Work out the finished part from the listing and answer in its coordinate system (mm). A direction names the side the tool comes from. Round coordinates to 2 decimals unless told otherwise and drop trailing zeros. Write each loop counter-clockwise with the first axis right and the second up, starting at its lowest first coordinate (ties: lowest second). Pieces come first, ordered by that corner, then holes.
from build123d import *

# Parameters (mm, degrees)
F0_R     = 1.6
F1_DEPTH = 7.5
F2_DEPTH = 50
F3_R     = 4
F4_DEPTH = 59.0844929405


with BuildPart() as f1:
    # F0 (on Top) → F1 (new body, symmetric)
    with BuildSketch(Plane.XY):
        Polygon((-5.0834929405, -4.2403818204), (-5.0834929405, -22.2403818204), (4, -30.0603818204), (4, 1.7596181796), align=None)
        with Locations((0, -19.8643818204)):
            Circle(F0_R, mode=Mode.SUBTRACT)
        with Locations((-0.412, -7.8643818204)):
            Circle(F0_R, mode=Mode.SUBTRACT)
    extrude(amount=F1_DEPTH, both=True)

    # F2 (add): a face of the model
    f2_faces = [f1.faces().sort_by_distance(p)[0] for p in [
        (-5.0834929405, -13.2403818204, 0),
    ]]
    extrude(f2_faces, amount=F2_DEPTH)

    # F3 (on face) → F4 (cut, through all)
    with BuildSketch(Plane.YZ.offset(4)):
        with Locations((-14.1503818204, 0)):
            Circle(F3_R)
    extrude(amount=-F4_DEPTH, mode=Mode.SUBTRACT)


solid = f1.part
Q1. Find the intervals of material crossed by L1, parallel to Y at x = -37, z = 0.25; L2, parallel to Y at x = -1, z = 3.25; L3, parallel to Y at x = -34.5, z = -1, in increasing order.
Q2. Find section D-D (x = 0). Determine the outline of the cut face in (y, z), plus the area to 3 significant figures.
Q3. Find section A-A (z = 0). Determine the outline of the cut face in (x, y).
Q4. A tool of negligible diameter and unlimited length cuts with its end or side. For faces 5 (the face through (-25, -14, -7.5)), 6 (the face through (-30, -4.24, 0)), from which of +Z, -Z, +X, -X, +Y, -Y can it reach the whole face along a straight path? Write none if from no direction.
Q5. Find section B-B (x = -35). Determine the outline of the cut face in (y, z), plus the area to 3 significant figures.
Q6. Find section C-C (y = -16). Determine the outline of the cut face in (x, z).
Q7. Given pin 1 (8 mm diameter, centred on x = -6, z = -4, fed in from +Y); pin 2 (4.5 mm diameter, centred on x = -22, z = 0, fed in from +Y); pin 3 (2.5 mm diameter, centred on x = -0.41, y = -7.86, fed in from -Z); pin 4 (7.5 mm diameter, centred on x = -29, z = -2, fed in from -Y), each flat-ended and moving along its own axis, determine where each tip first touches the part or whether it passes through.
Q8. The mould has two halves that part along X. Classify faces 1 (the face through (0.86, -18.515, -0.105)), 2 (the face through (4, -18, 2)), 3 (the face through (-30, -22.24, 0)), 4 (the face through (-55.083, -9, 0)): +X half, -X half, draft (parallel to the pull), parting line (faces both ways), or undercut.
Report:
1. L1: y = -22.24 to -18.14, -10.16 to -4.24
1. L2: y = -25.76 to -21.11, -18.62 to -16.48, -11.82 to -9.35, -6.38 to -1.54
1. L3: y = -22.24 to -18.02, -10.28 to -4.24
2. outline: (-26.62, -7.5) - (-21.46, -7.5) - (-21.46, 7.5) - (-26.62, 7.5) - close; (-18.26, -7.5) - (-9.41, -7.5) - (-9.41, 7.5) - (-18.26, 7.5) - close; (-6.32, -7.5) - (-0.88, -7.5) - (-0.88, 7.5) - (-6.32, 7.5) - close; hole circle Ø8 at (-14.15, 0)
2. area: 241 mm2
3. outline: (-55.08, -22.24) - (-5.08, -22.24) - (4, -30.06) - (4, -18.15) - (-55.08, -18.15) - close; (-55.08, -10.15) - (4, -10.15) - (4, 1.76) - (-5.08, -4.24) - (-55.08, -4.24) - close; hole circle Ø3.2 at (-0.41, -7.86); hole circle Ø3.2 at (0, -19.86)
4. face 5: -Z, +X, -X, +Y, -Y
4. face 6: +Z, -Z, -X, +Y
5. outline: (-22.24, -7.5) - (-4.24, -7.5) - (-4.24, 7.5) - (-22.24, 7.5) - close; hole circle Ø8 at (-14.15, 0)
5. area: 220 mm2
6. outline: (-55.08, -7.5) - (4, -7.5) - (4, -3.55) - (-55.08, -3.55) - close; (-55.08, 3.55) - (4, 3.55) - (4, 7.5) - (-55.08, 7.5) - close
7. pin 1: stops at y = -2.2
7. pin 2: stops at y = -4.24
7. pin 3: passes through
7. pin 4: stops at y = -22.24
8. face 1: undercut
8. face 2: +X half
8. face 3: draft
8. face 4: -X half
